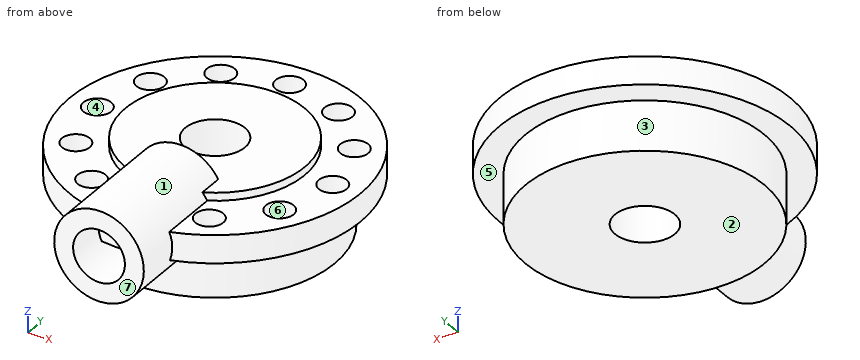
from build123d import *

# Parameters (mm, degrees)
SKETCH1_R                = 60
BOSS_EXTRUDE1_DEPTH      = 25
SKETCH2_R                = 73
BOSS_EXTRUDE2_DEPTH      = 14
SKETCH4_R                = 45
BOSS_EXTRUDE3_DEPTH      = 4
SKETCH5_R                = 15
CUT_EXTRUDE1_DEPTH       = 99
SKETCH6_R                = 7
CUT_EXTRUDE2_DEPTH       = 10
BOSS_EXTRUDE4_DEPTH      = 19
BOSS_EXTRUDE4_DEPTH_BACK = 45
SKETCH7_R                = 22.5
SKETCH7_R_2              = 13


with BuildPart() as part:
    # Sketch1 → Boss-Extrude1 (new body)
    with BuildSketch(Plane.XY):
        Circle(SKETCH1_R)
    extrude(amount=BOSS_EXTRUDE1_DEPTH)

    # Sketch2 → Boss-Extrude2 (add)
    with BuildSketch(Plane.XY.offset(25)):
        with Locations(Location((0, 0, 0), (0, 0, 180))):
            Circle(SKETCH2_R)
    extrude(amount=BOSS_EXTRUDE2_DEPTH)

    # Sketch4 → Boss-Extrude3 (add)
    with BuildSketch(Plane.XY.offset(39)):
        Circle(SKETCH4_R)
    extrude(amount=BOSS_EXTRUDE3_DEPTH)

    # Sketch5 → Cut-Extrude1 (cut)
    with BuildSketch(Plane.XY.offset(43)):
        Circle(SKETCH5_R)
    extrude(amount=-CUT_EXTRUDE1_DEPTH, mode=Mode.SUBTRACT)

    # Sketch6 → Cut-Extrude2 (cut)
    with BuildSketch(Plane.XY.offset(39)):
        with Locations((0, 59.095126961)):
            Circle(SKETCH6_R)
        with Locations((29.54756348, 51.177881188)):
            Circle(SKETCH6_R)
        with Locations((51.177881188, 29.54756348)):
            Circle(SKETCH6_R)
        with Locations((59.095126961, 0)):
            Circle(SKETCH6_R)
        with Locations((51.177881188, -29.54756348)):
            Circle(SKETCH6_R)
        with Locations((29.54756348, -51.177881188)):
            Circle(SKETCH6_R)
        with Locations((-29.54756348, -51.177881188)):
            Circle(SKETCH6_R)
        with Locations((-51.177881188, -29.54756348)):
            Circle(SKETCH6_R)
        with Locations((-59.095126961, 0)):
            Circle(SKETCH6_R)
        with Locations((-51.177881188, 29.54756348)):
            Circle(SKETCH6_R)
        with Locations((-29.54756348, 51.177881188)):
            Circle(SKETCH6_R)
    extrude(amount=-CUT_EXTRUDE2_DEPTH, mode=Mode.SUBTRACT)

    # Sketch7 → Boss-Extrude4 (add, two sides: drawn at the far end of the back side and taken through both)
    with BuildSketch(Plane(origin=(0, -73, 0), x_dir=(-1, 0, 0), z_dir=(0, -1, 0)).offset(-BOSS_EXTRUDE4_DEPTH_BACK)):
        with Locations(Location((0, -31.497185576, 0), (0, 0, 210.74620731))):
            Circle(SKETCH7_R)
        with Locations(Location((0, -31.497185576, 0), (0, 0, 297.769160661))):
            Circle(SKETCH7_R_2, mode=Mode.SUBTRACT)
    extrude(amount=BOSS_EXTRUDE4_DEPTH + BOSS_EXTRUDE4_DEPTH_BACK)


solid = part.part
Here's how the part is built. I have some questions about the finished solid (model axes, mm). Face numbers are marked on the shaded views. A direction names the side the tool comes from. Round coordinates to 2 decimals unless told otherwise and drop trailing zeros. Order: outer loops, then holes, each group sorted by start corner. A loop starts at its lowest first (then second) coordinate and runs counter-clockwise, first axis right, second up. Notation, with made-up numbers: (77.5, -0.75) -> (105.5, -0.75) arc R17 cw to (105.5, 20.25) -> close; hole circle Ø3 at (40, 43). An arc over 180 degrees is marked (long way). Return JSON: item names as keys, results as strings.
Q1. If we mould it in two halves opening along Y, with no side actions, what happens to the marked faces 5, 6 and 7? For each: released by +Y, released by -Y, zero draft, split by the parting line, or undercut.
Filled sheet:
{"face 5": "zero draft", "face 6": "undercut", "face 7": "released by -Y"}
Q2. If we section it at A-A on x = 0: List the corners of the cut face in (y, z) for me, plus the area to 3 significant figures.
Filled sheet:
{"outline": "(-92, 9) -> (-60, 9) -> (-60, 0) -> (-15, 0) -> (-15, 43) -> (-45, 43) -> (-45, 39) -> (-73, 39) -> (-73, 25) -> (-60, 25) -> (-60, 18.5) -> (-92, 18.5) -> close; (-92, 44.5) -> (-28, 44.5) -> (-28, 54) -> (-92, 54) -> close; (15, 0) -> (60, 0) -> (60, 25) -> (73, 25) -> (73, 39) -> (66.1, 39) -> (66.1, 29) -> (52.1, 29) -> (52.1, 39) -> (45, 39) -> (45, 43) -> (15, 43) -> close", "area": "4,890 mm^2"}
Q3. For pin 1 Ø6.5 at (x, y) = (-4, -51.5) entering from +Z; pin 2 Ø15.5 at (x, y) = (61.5, -3) entering from +Z; pin 3 Ø3 at (x, z) = (47.5, 36.5) entering from +Y; pin 4 Ø8.5 at (x, y) = (29.55, -51.18) entering from -Z, each with a flat end and sliding along its axis, tell me the tip position at first contact or that it passes through.
Filled sheet:
{"pin 1": "stops at z = 53.98", "pin 2": "stops at z = 39", "pin 3": "stops at y = 56.68", "pin 4": "stops at z = 0"}
Q4. If we section it at B-B on y = 0: List the corners of the cut face in (x, z) for me.
Filled sheet:
{"outline": "(-73, 25) -> (-60, 25) -> (-60, 0) -> (-15, 0) -> (-15, 43) -> (-45, 43) -> (-45, 39) -> (-52.1, 39) -> (-52.1, 29) -> (-66.1, 29) -> (-66.1, 39) -> (-73, 39) -> close; (15, 0) -> (60, 0) -> (60, 25) -> (73, 25) -> (73, 39) -> (66.1, 39) -> (66.1, 29) -> (52.1, 29) -> (52.1, 39) -> (45, 39) -> (45, 43) -> (15, 43) -> close"}
Q5. If we section it at D-D on x = 26: List the corners of the cut face in (y, z) for me, plus the area to 3 significant figures.
Filled sheet:
{"outline": "(-68.21, 25) -> (-54.07, 25) -> (-54.07, 0) -> (54.07, 0) -> (54.07, 25) -> (68.21, 25) -> (68.21, 39) -> (57.21, 39) -> (57.21, 29) -> (45.14, 29) -> (45.14, 39) -> (36.73, 39) -> (36.73, 43) -> (-36.73, 43) -> (-36.73, 39) -> (-45.14, 39) -> (-45.14, 29) -> (-57.21, 29) -> (-57.21, 39) -> (-68.21, 39) -> close", "area": "4,670 mm^2"}
Q6. Which directions (+Z, -Z, +X, -X, +Y, -Y) give clear straight access to the entire face, cutting with the end or side of a thin tool? Please do the marked faces 1, 2, 3 and 4.
Filled sheet:
{"face 1": "-Y", "face 2": "-Z, +X, -X, +Y, -Y", "face 3": "-Z", "face 4": "+Z"}
Q7. If we section it at C-C on z = 15: List the corners of the cut face in (x, y) for me, plus the area to 3 significant figures.
Filled sheet:
{"outline": "(-15.3, -92) -> (15.3, -92) -> (15.3, -58.02) arc R60 ccw (long way) to (-15.3, -58.02) -> close; hole circle Ø30 at (0, 0)", "area": "11,600 mm^2"}
Q8. I need wall thicknesses on line 1 along Y through (x, z) = (1, 34); line 2 along Z through (x, y) = (21.5, -2); line 3 along X through (y, z) = (-7.5, 21). Which ranges of each line are inside material? Lowest first, please. Write a range as from..to.
Filled sheet:
{"line 1": "y = -72.99..-14.97, 14.97..52.17, 66.02..72.99", "line 2": "z = 0..43", "line 3": "x = -59.53..-12.99, 12.99..59.53"}
